```python
from build123d import *

# Parameters (mm, degrees)
SKETCH1_W           = 132.221839449
SKETCH1_H           = 62.399911756
BOSS_EXTRUDE1_DEPTH = 5
SKETCH2_R           = 4
BOSS_EXTRUDE2_DEPTH = 15


with BuildPart() as part:
    # Sketch1 → Boss-Extrude1 (new body)
    with BuildSketch(Plane.XY):
        with Locations((10.583244946, -0.274889479)):
            Rectangle(SKETCH1_W, SKETCH1_H)
    extrude(amount=BOSS_EXTRUDE1_DEPTH)

    # Sketch2 → Boss-Extrude2 (add)
    with BuildSketch(Plane.XY.offset(5)):
        with Locations((-18.035961804, -0.274889479)):
            Circle(SKETCH2_R)
        with Locations(Location((39.202451695, -0.274889479, 0), (0, 0, 180))):
            Circle(SKETCH2_R)
    extrude(amount=BOSS_EXTRUDE2_DEPTH)


solid = part.part
```
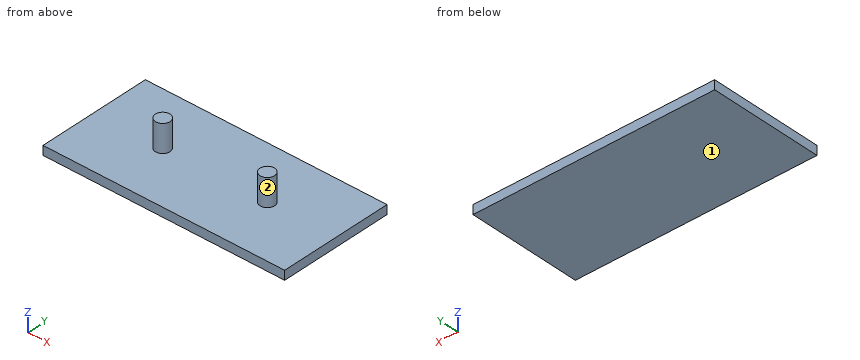
Could you check a few things on this model? Use its own coordinates, in mm. Face numbers are marked on the shaded views. Give positions to 0.01 mm unless a question says otherwise; leave off trailing zeros. Loops run counter-clockwise (first coordinate to the right, second up) from the corner with the lowest first, then second, coordinate; pieces in that order, holes last. Notation, with made-up numbers: (51.25, 43) -> (55.25, 43) arc R32 ccw to (55.25, 78) -> close; hole circle Ø11 at (-12, -22). An arc over 180 degrees is marked (long way). Put each result on its own line as item: value.
(1) I'm going to push flat-ended pins straight in: pin 1 Ø3 at (x, y) = (42.5, 16.5) entering from +Z; pin 2 Ø12 at (y, z) = (10, 15) entering from +X. Where does each tip first touch, or does it pass through?
Computed:
pin 1: z = 5
pin 2: through
(2) Thinking about a two-plate mould opening in X: for the marked faces 1 and 2, which applies, pulls with the +X half, pulls with the -X half, needs draft (parallel to the pull), parting line crosses it, or undercut?
Computed:
face 1: needs draft
face 2: undercut
(3) Imagine slicing it at A-A on y = 16. Write out the boundary of the cut face in (x, z), plus the area to 3 significant figures.
Computed:
outline: (-55.53, 0) -> (76.69, 0) -> (76.69, 5) -> (-55.53, 5) -> close
area: 661 mm^2
(4) Imagine slicing it at B-B on x = -16. Write out the boundary of the cut face in (y, z).
Computed:
outline: (-31.47, 0) -> (30.93, 0) -> (30.93, 5) -> (3.17, 5) -> (3.17, 20) -> (-3.72, 20) -> (-3.72, 5) -> (-31.47, 5) -> close
(5) Please list where these lines run through material, in increasing order: probe 1 along X at (y, z) = (0, 5.5); probe 2 along Z at (x, y) = (-21, -28); probe 3 along Y at (x, z) = (-15.5, 15). Write a range as [from, to].
Computed:
probe 1: [-22.03, -14.05], [35.21, 43.19]
probe 2: [0, 5]
probe 3: [-3.37, 2.82]
(6) Imagine slicing it at C-C on z = 17. Write out the boundary of the cut face in (x, y).
Computed:
outline: circle Ø8 at (-18.04, -0.27); circle Ø8 at (39.2, -0.27)
(7) Imagine slicing it at D-D on y = -2. Write out the boundary of the cut face in (x, z), plus the area to 3 significant figures.
Computed:
outline: (-55.53, 0) -> (76.69, 0) -> (76.69, 5) -> (42.81, 5) -> (42.81, 20) -> (35.59, 20) -> (35.59, 5) -> (-14.43, 5) -> (-14.43, 20) -> (-21.64, 20) -> (-21.64, 5) -> (-55.53, 5) -> close
area: 878 mm^2
